```python
from build123d import *

# Parameters (mm, degrees)
SKETCH_1_R          = 18.5
EXTRUDE_1_DEPTH     = 24
SKETCH_2_R          = 16.5
EXTRUDE_2_DEPTH     = 32
SKETCH_4_R          = 1.5
CUT_EXTRUDE_1_DEPTH = 6
SKETCH_5_R          = 6
EXTRUDE_3_DEPTH     = 6
EXTRUDE_4_DEPTH     = 12
EXTRUDE_5_DEPTH     = 6


with BuildPart() as part:
    # 草图1 → 凸台-拉伸1 (new body)
    with BuildSketch(Plane(origin=(0, 0, 0), x_dir=(0, 0, -1), z_dir=(1, 0, 0))):
        Circle(SKETCH_1_R)
    extrude(amount=EXTRUDE_1_DEPTH)

    # 草图2 → 凸台-拉伸2 (add)
    with BuildSketch(Plane.ZY):
        Circle(SKETCH_2_R)
    extrude(amount=EXTRUDE_2_DEPTH)

    # 草图4 → 切除-拉伸1 (cut)
    with BuildSketch(Plane(origin=(24, 0, 0), x_dir=(0, 0, -1), z_dir=(1, 0, 0))):
        with Locations((15.5, 0)):
            Circle(SKETCH_4_R)
        with Locations((7.75, -13.423393759)):
            Circle(SKETCH_4_R)
        with Locations((-7.75, -13.423393759)):
            Circle(SKETCH_4_R)
        with Locations((-15.5, 0)):
            Circle(SKETCH_4_R)
        with Locations((-7.75, 13.423393759)):
            Circle(SKETCH_4_R)
        with Locations((7.75, 13.423393759)):
            Circle(SKETCH_4_R)
    extrude(amount=-CUT_EXTRUDE_1_DEPTH, mode=Mode.SUBTRACT)

    # 草图5 → 凸台-拉伸3 (add)
    with BuildSketch(Plane(origin=(24, 0, 0), x_dir=(0, 0, -1), z_dir=(1, 0, 0))):
        with Locations((0, 7)):
            Circle(SKETCH_5_R)
    extrude(amount=EXTRUDE_3_DEPTH)

    # 草图6 → 凸台-拉伸4 (add)
    with BuildSketch(Plane(origin=(30, 0, 0), x_dir=(0, 0, -1), z_dir=(1, 0, 0))):
        with BuildLine():
            Line((-1.658312395, 9.5), (1.658312395, 9.5))
            ThreePointArc((1.658312395, 9.5), (0, 4), (-1.658312395, 9.5))
        make_face()
    extrude(amount=EXTRUDE_4_DEPTH)

    # 草图7 → 凸台-拉伸5 (add)
    with BuildSketch(Plane.ZY.offset(32)):
        Polygon((7.680859807, -20.274157757), (20.216755747, -7.8307003), (16.086686091, -3.669949673), (3.550790151, -16.113407129), align=None)
    extrude(amount=-EXTRUDE_5_DEPTH)


solid = part.part
```
The listing builds one solid part. Answer for the finished solid, in the listing's coordinates (mm). A direction names the side the tool comes from. Round coordinates to 2 decimals unless told otherwise and drop trailing zeros. Order: outer loops, then holes, each group sorted by start corner. A loop starts at its lowest first (then second) coordinate and runs counter-clockwise, first axis right, second up. Notation, with made-up numbers: (60, 22) - (97, 22) arc R29 ccw to (97, 52) - close; hole circle Ø6 at (32.5, -20.75). An arc over 180 degrees is marked (long way). Put each result on its own line as item: value. Start each with the question number.
(1) For faces 4 (the flat face through (0, 0, 17)), 5 (the flat face through (36, 9.5, 0)), 6 (the cylindrical face through (21.042, -12.41, -6.644)), determine the directions among +Z, -Z, +X, -X, +Y, -Y from which every point of the face is accessible in a straight line to the end or side of a thin tool.
(2) Find section B-B (x = 22). Give the vertices of the cut face in (y, z).
(3) Determine the mould class of faces 1 (the flat face through (-29, -14, 14)), 2 (the flat face through (18, 13, -8)), 3 (the flat face through (-26, -13, 12)) for opening direction Z: released by +Z, released by -Z, zero draft, split by the parting line, or undercut.
(4) Given P1, Ø10, axis at x = 7, y = -4, coming from the +Z side; P2, Ø1, axis at x = 3.5, y = -10.5, coming from the +Z side; P3, Ø3.5, axis at y = -0.5, z = 16, coming from the +X side, each flat-ended and moving along its own axis, determine where each tip first touches the part or whether it passes through.
(5) Straight lines are drawn through the part: probe 1 along X at (y, z) = (-5, 16); probe 2 along Y at (x, z) = (20, 7.75); probe 3 along X at (y, z) = (16, -6). For each, find the intervals that lie inside material, in ascending order. Write a range as from..to.
(6) Find section D-D (x = -8). Give the vertices of the cut face in (y, z), plus the area to 3 significant figures.
(7) Find section C-C (y = 0). Give the vertices of the cut face in (x, z), plus the area to 3 significant figures.
(8) Find section A-A (z = 0). Give the vertices of the cut face in (x, y).
Reply:
1. face 4: none
1. face 5: +Z, -Z, +X, +Y
1. face 6: +X
2. outline: circle Ø37 at (0, 0); hole circle Ø3 at (-13.42, -7.75); hole circle Ø3 at (-13.42, 7.75); hole circle Ø3 at (0, -15.5); hole circle Ø3 at (0, 15.5); hole circle Ø3 at (13.42, -7.75); hole circle Ø3 at (13.42, 7.75)
3. face 1: released by +Z
3. face 2: undercut
3. face 3: zero draft
4. P1: z = 18.5
4. P2: z = 15.56
4. P3: x = 24
5. probe 1: -32..-26, 0..24
5. probe 2: -16.8..-14.92, -11.92..11.92, 14.92..16.8
5. probe 3: 0..24
6. outline: circle Ø33 at (0, 0)
6. area: 855 mm^2
7. outline: (-32, -16.5) - (0, -16.5) - (0, -18.5) - (24, -18.5) - (24, -17) - (18, -17) - (18, -14) - (24, -14) - (24, 14) - (18, 14) - (18, 17) - (24, 17) - (24, 18.5) - (0, 18.5) - (0, 16.5) - (-32, 16.5) - close
7. area: 1,910 mm^2
8. outline: (-32, -16.5) - (0, -16.5) - (0, -18.5) - (24, -18.5) - (24, 1) - (30, 1) - (30, 4) - (42, 4) - (42, 9.5) - (30, 9.5) - (30, 13) - (24, 13) - (24, 18.5) - (0, 18.5) - (0, 16.5) - (-32, 16.5) - close
